from build123d import *
from OCP.BRepFilletAPI import BRepFilletAPI_MakeChamfer

# Parameters (mm, degrees)
EXTRUDE2_DEPTH     = 8
CHAMFER2_SIZE      = 4
CHAMFER2_SIZE2     = 2.309401077
CUT_EXTRUDE1_DEPTH = 3
EXTRUDE3_START     = 8
EXTRUDE3_DEPTH     = 40
SKETCH4_R          = 3.05
CUT_EXTRUDE2_DEPTH = 78.989993783
FILLET1_R          = 1


with BuildPart() as part:
    # Sketch1 → Extrude2 (new body)
    with BuildSketch(Plane(origin=(0, 0, 0), x_dir=(1, 0, 0), z_dir=(0, 1, 0))):
        with BuildLine():
            Line((-6.5, 41.572883869), (-16.221725084, 16.871170844))
            ThreePointArc((-16.221725084, 16.871170844), (-17.527996386, 13.882959965), (-19.052558883, 11))
            ThreePointArc((-19.052558883, 11), (-20.786994202, 8.238210165), (-22.721725084, 5.612840594))
            Line((-22.721725084, 5.612840594), (-39.253173539, -15.15727681))
            ThreePointArc((-39.253173539, -15.15727681), (-39.837168574, -23), (-32.753173539, -26.415607059))
            Line((-32.753173539, -26.415607059), (-6.5, -22.484011438))
            ThreePointArc((-6.5, -22.484011438), (-3.258997817, -22.12117013), (0, -22))
            ThreePointArc((0, -22), (3.258997817, -22.12117013), (6.5, -22.484011438))
            Line((6.5, -22.484011438), (32.753173539, -26.415607059))
            ThreePointArc((32.753173539, -26.415607059), (39.837168574, -23), (39.253173539, -15.15727681))
            Line((39.253173539, -15.15727681), (22.721725084, 5.612840594))
            ThreePointArc((22.721725084, 5.612840594), (20.786994202, 8.238210165), (19.052558883, 11))
            ThreePointArc((19.052558883, 11), (17.527996386, 13.882959965), (16.221725084, 16.871170844))
            Line((16.221725084, 16.871170844), (6.5, 41.572883869))
            ThreePointArc((6.5, 41.572883869), (0, 46), (-6.5, 41.572883869))
        make_face()
    extrude(amount=EXTRUDE2_DEPTH)

    # Chamfer2: one chamfer whose edges measure the first distance from different faces: ONE call of the kernel's chamfer builder (chamfer() names one face for all edges)
    chamfer2_edges_1 = [part.edges().sort_by_distance(p)[0] for p in [
        (-19.052558883, 8, -11),
    ]]
    chamfer2_side_1 = [part.faces().sort_by_distance(p)[0] for p in [
        (-19.052558883, 4, -11),
    ]]
    chamfer2_edges_2 = [part.edges().sort_by_distance(p)[0] for p in [
        (-30.987449312, 8, 4.772218108),
    ]]
    chamfer2_side_2 = [part.faces().sort_by_distance(p)[0] for p in [
        (-30.987449312, 4, 4.772218108),
    ]]
    chamfer2_edges_3 = [part.edges().sort_by_distance(p)[0] for p in [
        (-39.837168574, 8, 23),
    ]]
    chamfer2_side_3 = [part.faces().sort_by_distance(p)[0] for p in [
        (-39.837168574, 4, 23),
    ]]
    chamfer2_edges_4 = [part.edges().sort_by_distance(p)[0] for p in [
        (-19.626586769, 8, 24.449809248),
    ]]
    chamfer2_side_4 = [part.faces().sort_by_distance(p)[0] for p in [
        (-19.626586769, 4, 24.449809248),
    ]]
    chamfer2_edges_5 = [part.edges().sort_by_distance(p)[0] for p in [
        (0, 8, 22),
    ]]
    chamfer2_side_5 = [part.faces().sort_by_distance(p)[0] for p in [
        (0, 4, 22),
    ]]
    chamfer2_edges_6 = [part.edges().sort_by_distance(p)[0] for p in [
        (19.626586769, 8, 24.449809248),
    ]]
    chamfer2_side_6 = [part.faces().sort_by_distance(p)[0] for p in [
        (19.626586769, 4, 24.449809248),
    ]]
    chamfer2_edges_7 = [part.edges().sort_by_distance(p)[0] for p in [
        (39.837168574, 8, 23),
    ]]
    chamfer2_side_7 = [part.faces().sort_by_distance(p)[0] for p in [
        (39.837168574, 4, 23),
    ]]
    chamfer2_edges_8 = [part.edges().sort_by_distance(p)[0] for p in [
        (30.987449312, 8, 4.772218108),
    ]]
    chamfer2_side_8 = [part.faces().sort_by_distance(p)[0] for p in [
        (30.987449312, 4, 4.772218108),
    ]]
    chamfer2_edges_9 = [part.edges().sort_by_distance(p)[0] for p in [
        (0, 8, -46),
    ]]
    chamfer2_side_9 = [part.faces().sort_by_distance(p)[0] for p in [
        (0, 4, -46),
    ]]
    chamfer2_edges_10 = [part.edges().sort_by_distance(p)[0] for p in [
        (19.052558883, 8, -11),
    ]]
    chamfer2_side_10 = [part.faces().sort_by_distance(p)[0] for p in [
        (19.052558883, 4, -11),
    ]]
    chamfer2_edges_11 = [part.edges().sort_by_distance(p)[0] for p in [
        (11.360862542, 8, -29.222027356),
    ]]
    chamfer2_side_11 = [part.faces().sort_by_distance(p)[0] for p in [
        (11.360862542, 4, -29.222027356),
    ]]
    chamfer2_edges_12 = [part.edges().sort_by_distance(p)[0] for p in [
        (-11.360862542, 8, -29.222027356),
    ]]
    chamfer2_side_12 = [part.faces().sort_by_distance(p)[0] for p in [
        (-11.360862542, 4, -29.222027356),
    ]]
    chamfer2 = BRepFilletAPI_MakeChamfer(part.part.solid().wrapped)
    for e in chamfer2_edges_1:
        chamfer2.Add(CHAMFER2_SIZE, CHAMFER2_SIZE2, e.wrapped, chamfer2_side_1[0].wrapped)  # the first distance lies on this face
    for e in chamfer2_edges_2:
        chamfer2.Add(CHAMFER2_SIZE, CHAMFER2_SIZE2, e.wrapped, chamfer2_side_2[0].wrapped)  # the first distance lies on this face
    for e in chamfer2_edges_3:
        chamfer2.Add(CHAMFER2_SIZE, CHAMFER2_SIZE2, e.wrapped, chamfer2_side_3[0].wrapped)  # the first distance lies on this face
    for e in chamfer2_edges_4:
        chamfer2.Add(CHAMFER2_SIZE, CHAMFER2_SIZE2, e.wrapped, chamfer2_side_4[0].wrapped)  # the first distance lies on this face
    for e in chamfer2_edges_5:
        chamfer2.Add(CHAMFER2_SIZE, CHAMFER2_SIZE2, e.wrapped, chamfer2_side_5[0].wrapped)  # the first distance lies on this face
    for e in chamfer2_edges_6:
        chamfer2.Add(CHAMFER2_SIZE, CHAMFER2_SIZE2, e.wrapped, chamfer2_side_6[0].wrapped)  # the first distance lies on this face
    for e in chamfer2_edges_7:
        chamfer2.Add(CHAMFER2_SIZE, CHAMFER2_SIZE2, e.wrapped, chamfer2_side_7[0].wrapped)  # the first distance lies on this face
    for e in chamfer2_edges_8:
        chamfer2.Add(CHAMFER2_SIZE, CHAMFER2_SIZE2, e.wrapped, chamfer2_side_8[0].wrapped)  # the first distance lies on this face
    for e in chamfer2_edges_9:
        chamfer2.Add(CHAMFER2_SIZE, CHAMFER2_SIZE2, e.wrapped, chamfer2_side_9[0].wrapped)  # the first distance lies on this face
    for e in chamfer2_edges_10:
        chamfer2.Add(CHAMFER2_SIZE, CHAMFER2_SIZE2, e.wrapped, chamfer2_side_10[0].wrapped)  # the first distance lies on this face
    for e in chamfer2_edges_11:
        chamfer2.Add(CHAMFER2_SIZE, CHAMFER2_SIZE2, e.wrapped, chamfer2_side_11[0].wrapped)  # the first distance lies on this face
    for e in chamfer2_edges_12:
        chamfer2.Add(CHAMFER2_SIZE, CHAMFER2_SIZE2, e.wrapped, chamfer2_side_12[0].wrapped)  # the first distance lies on this face
    add(Compound.cast(chamfer2.Shape()), mode=Mode.REPLACE)

    # Sketch2 → Cut-Extrude1 (cut)
    with BuildSketch(Plane(origin=(0, 0, 0), x_dir=(1, 0, 0), z_dir=(0, 1, 0))):
        with BuildLine():
            ThreePointArc((-33.06983816, -24.960303026), (-38.550871935, -22.25735629), (-38.151175585, -16.159168435))
            ThreePointArc((-38.151175585, -16.159168435), (-36.048003444, -15.88228057), (-35.771115574, -17.985452713))
            ThreePointArc((-35.771115574, -17.985452713), (-35.952795735, -20.757356297), (-33.461416734, -21.985968456))
            ThreePointArc((-33.461416734, -21.985968456), (-31.778460163, -23.277346457), (-33.06983816, -24.960303026))
        make_face()
        with BuildLine():
            ThreePointArc((-5.081337427, 41.119471458), (0, 44.514712578), (5.081337424, 41.119471458))
            ThreePointArc((5.081337424, 41.119471458), (4.269543279, 39.159627023), (2.309698839, 39.971421166))
            ThreePointArc((2.309698839, 39.971421166), (0, 41.514712592), (-2.309698842, 39.971421166))
            ThreePointArc((-2.309698842, 39.971421166), (-4.269543282, 39.159627023), (-5.081337427, 41.119471458))
        make_face()
        with BuildLine():
            ThreePointArc((38.151175587, -16.159168432), (38.550871936, -22.257356289), (33.069838162, -24.960303024))
            ThreePointArc((33.069838162, -24.960303024), (31.778460165, -23.277346454), (33.461416736, -21.985968453))
            ThreePointArc((33.461416736, -21.985968453), (35.952795736, -20.757356296), (35.771115577, -17.985452711))
            ThreePointArc((35.771115577, -17.985452711), (36.048003446, -15.882280567), (38.151175587, -16.159168432))
        make_face()
    extrude(amount=CUT_EXTRUDE1_DEPTH, mode=Mode.SUBTRACT)

    # Sketch3 → Extrude3 (add)
    with BuildSketch(Plane(origin=(0, 0, 0), x_dir=(1, 0, 0), z_dir=(0, 1, 0)).offset(EXTRUDE3_START)):
        with BuildLine():
            Line((-20, 0), (-20, -10))
            Line((-20, -10), (20, -10))
            Line((20, -10), (20, 0))
            Line((20, 0), (3.5, 0))
            ThreePointArc((3.5, 0), (0, -3.5), (-3.5, 0))
            Line((-3.5, 0), (-20, 0))
        make_face()
    extrude(amount=EXTRUDE3_DEPTH)

    # Sketch4 → Cut-Extrude2 (cut, through all)
    with BuildSketch(Plane.XY):
        with Locations(Location((-12.5, 40.5, 0), (0, 0, 180))):
            Circle(SKETCH4_R)
        with Locations(Location((12.5, 40.5, 0), (0, 0, 180))):
            Circle(SKETCH4_R)
        with Locations(Location((12.5, 15.5, 0), (0, 0, 180))):
            Circle(SKETCH4_R)
        with Locations(Location((-12.5, 15.5, 0), (0, 0, 180))):
            Circle(SKETCH4_R)
    extrude(amount=CUT_EXTRUDE2_DEPTH, mode=Mode.SUBTRACT)

    # Fillet1
    fillet1_edges = [part.edges().sort_by_distance(p)[0] for p in [
        (-20, 8, 5),
        (11.360862542, 0, -29.222027356),
        (0, 8, 10),
        (-20, 28, 10),
        (20, 8, 5),
        (20, 28, 10),
        (-20, 48, 5),
        (0, 48, 10),
        (20, 48, 5),
        (19.052558883, 0, -11),
        (30.987449312, 0, 4.772218108),
        (39.837168574, 0, 23),
        (19.626586769, 0, 24.449809248),
        (0, 0, 22),
        (-19.626586769, 0, 24.449809248),
        (-39.837168574, 0, 23),
        (-30.987449312, 0, 4.772218108),
        (-19.052558883, 0, -11),
        (-11.360862542, 0, -29.222027356),
        (0, 0, -46),
    ]]
    fillet(fillet1_edges, radius=FILLET1_R)


solid = part.part
Read the model definition and answer for the solid it produces. Units are mm, in the model's axes. A direction names the side the tool comes from. Give positions to 0.01 mm unless a question says otherwise; leave off trailing zeros. Loops run counter-clockwise (first coordinate to the right, second up) from the corner with the lowest first, then second, coordinate; pieces in that order, holes last. Notation, with made-up numbers: (-22, 89.5) -> (-12, 89.5) arc R19 ccw to (-12, 104.5) -> close; hole circle Ø4 at (2.25, 38). An arc over 180 degrees is marked (long way). Answer as CSV lines item,"result".
Item 1: Consider line 1 (X direction, y = 40.5, z = 7); line 2 (Y direction, x = -12.5, z = 7.75); line 3 (Z direction, x = -11, y = 30). Determine where each line is inside the solid, lowest interval first. Write a range as [from, to].
Returned:
line 1,"x = [-20, -15.55], [-9.45, 9.45], [15.55, 20]"
line 2,"y = [0, 12.45], [18.55, 37.45], [43.55, 48]"
line 3,"z = [0, 10]"
Item 2: Find section C-C on x = 11. State how many separate pieces and enclosed holes the cut face has, plus the area to 3 significant figures.
Returned:
separate pieces,"3"
enclosed holes,"0"
area,"702 mm²"
Item 3: Find section A-A on y = 40.5. Give the vertices of the cut face in (x, z), plus the area to 3 significant figures.
Returned:
outline,"(-20, 0) -> (-15.55, 0) -> (-15.55, 10) -> (-19, 10) arc R1 ccw to (-20, 9) -> close; (-9.45, 0) -> (-3.5, 0) arc R3.5 cw to (3.5, 0) -> (9.45, 0) -> (9.45, 10) -> (-9.45, 10) -> close; (15.55, 0) -> (20, 0) -> (20, 9) arc R1 ccw to (19, 10) -> (15.55, 10) -> close"
area,"258 mm²"
Item 4: Determine the mould class of faces 5 (the face through (0, 2, -46)), 6 (the face through (4.3, 1.479, -39.173)), 7 (the face through (-39.895, 2.479, 22.898)) for opening direction Z: +Z half, -Z half, draft (parallel to the pull), parting line (faces both ways), or undercut.
Returned:
face 5,"-Z half"
face 6,"undercut"
face 7,"parting line"
Item 5: Each of these flat-tipped pins is pushed along its axis until it touches: pin 1 (5 mm diameter, centred on x = -12.5, y = 26.5, fed in from -Z); pin 2 (10 mm diameter, centred on x = -28, y = 10.5, fed in from -Z); pin 3 (10 mm diameter, centred on x = 11.5, z = -38, fed in from +Y); pin 4 (3 mm diameter, centred on x = -13, y = 40.5, fed in from -Z). Where does it stop, or does it pass through?
Returned:
pin 1,"stops at z = 0"
pin 2,"stops at z = -0.76"
pin 3,"stops at y = 6.87"
pin 4,"passes through"
Item 6: For faces 1 (the face through (-12, 28, 0)), 2 (the face through (20, 28, 5)), 3 (the face through (-19.984, 6.028, 23.319)), 4 (the face through (35.932, 1.479, 20.793)), determine the directions among +Z, -Z, +X, -X, +Y, -Y from which every point of the face is accessible in a straight line to the end or side of a thin tool.
Returned:
face 1,"-Z, +X, -X, +Y"
face 2,"+Z, -Z, +X, +Y"
face 3,"+Z, +Y"
face 4,"-Y"
Item 7: Find section B-B on y = 22. Give the vertices of the cut face in (x, z), plus the area to 3 significant figures.
Returned:
outline,"(-20, 0) -> (-3.5, 0) arc R3.5 cw to (3.5, 0) -> (20, 0) -> (20, 9) arc R1 ccw to (19, 10) -> (-19, 10) arc R1 ccw to (-20, 9) -> close"
area,"380 mm²"
